The model under review builds one solid part; all positions refer to its coordinate system, in mm. Give positions to 0.01 mm unless a question says otherwise; leave off trailing zeros. Order: outer loops, then holes, each group sorted by start corner. A loop starts at its lowest first (then second) coordinate and runs counter-clockwise, first axis right, second up. Notation, with made-up numbers: (63.5, -6.5) - (110.5, -6.5) arc R31 cw to (110.5, 24.5) - close; hole circle Ø5 at (-14.75, 3.25). An arc over 180 degrees is marked (long way). Write item = value, one per line. Start each with the question number.
1. Mouldability with a two-part tool opening along X and no side actions: class faces 1 (the cylindrical face through (20.797, -14.859, 3.219)), 2 (the flat face through (0, 16, 3)), 3 (the cylindrical face through (-19.31, -13, 3.22)), 4 (the cylindrical face through (-20.859, 14.797, 3.219)) as pulls with the +X half, pulls with the -X half, needs draft (parallel to the pull), parting line crosses it, or undercut.
2. We need section B-B, the plane y = -6. Give the boundary of the cut face in (x, z), and give its area (3 significant figures).
3. We need section C-C, the plane y = -13. Give the boundary of the cut face in (x, z), and give its area (3 significant figures).
4. For P1, Ø2, axis at x = -9.19, y = -9.19, coming from the +Z side (3 decimals), flat-tipped, find the tip position at first contact; note if it passes through.
5. Wall thickness on probe 1 along Y at (x, z) = (18, 3.5); probe 2 along X at (y, z) = (11.5, 3); probe 3 along X at (y, z) = (-8.5, 2.5): over which ranges is each line inside the solid? List them lowest first.
6. We need section A-A, the plane x = 0. Give the boundary of the cut face in (y, z), and give its area (4 significant figures).
7. We need section D-D, the plane x = -9. Give the boundary of the cut face in (y, z).
from build123d import *

# Parameters (mm, degrees)
SKETCH1_W           = 44
SKETCH1_H           = 32
SKETCH1_R           = 9.5
SKETCH1_R_2         = 1.65
BOSS_EXTRUDE1_DEPTH = 6.35
SKETCH2_R           = 1.65
CUT_EXTRUDE1_DEPTH  = 28.934253167
FILLET1_R           = 4


with BuildPart() as part:
    # Sketch1 → Boss-Extrude1 (new body)
    with BuildSketch(Plane.XY):
        Rectangle(SKETCH1_W, SKETCH1_H)
        Circle(SKETCH1_R, mode=Mode.SUBTRACT)
        with Locations((-9.192388155, 9.192388155)):
            Circle(SKETCH1_R_2, mode=Mode.SUBTRACT)
        with Locations((9.192388155, 9.192388155)):
            Circle(SKETCH1_R_2, mode=Mode.SUBTRACT)
        with Locations((9.192388155, -9.192388155)):
            Circle(SKETCH1_R_2, mode=Mode.SUBTRACT)
        with Locations((-9.192388155, -9.192388155)):
            Circle(SKETCH1_R_2, mode=Mode.SUBTRACT)
    extrude(amount=BOSS_EXTRUDE1_DEPTH)

    # Sketch2 → Cut-Extrude1 (cut, through all)
    with BuildSketch(Plane.XY.offset(6.35)):
        with Locations((-18, 12)):
            Circle(SKETCH2_R)
        with Locations((-18, -12)):
            Circle(SKETCH2_R)
        with Locations((18, -12)):
            Circle(SKETCH2_R)
        with Locations((18, 12)):
            Circle(SKETCH2_R)
    extrude(amount=-CUT_EXTRUDE1_DEPTH, mode=Mode.SUBTRACT)

    # Fillet1
    fillet1_edges = [part.edges().sort_by_distance(p)[0] for p in [
        (-22, 16, 3.175),
        (22, 16, 3.175),
        (22, -16, 3.175),
        (-22, -16, 3.175),
    ]]
    fillet(fillet1_edges, radius=FILLET1_R)


solid = part.part
Model answer:
q1.face_1 = pulls with the +X half
q1.face_2 = needs draft
q1.face_3 = undercut
q1.face_4 = pulls with the -X half
q2.outline = (-22, 0) - (-7.37, 0) - (-7.37, 6.35) - (-22, 6.35) - close; (7.37, 0) - (22, 0) - (22, 6.35) - (7.37, 6.35) - close
q2.area = 186 mm2
q3.outline = (-21.87, 0) - (-19.31, 0) - (-19.31, 6.35) - (-21.87, 6.35) - close; (-16.69, 0) - (16.69, 0) - (16.69, 6.35) - (-16.69, 6.35) - close; (19.31, 0) - (21.87, 0) - (21.87, 6.35) - (19.31, 6.35) - close
q3.area = 244 mm2
q4.P1 = through
q5.probe_1 = -16 to -13.65, -10.35 to 10.35, 13.65 to 16
q5.probe_2 = -22 to -19.57, -16.43 to 16.43, 19.57 to 22
q5.probe_3 = -22 to -10.69, -7.69 to -4.24, 4.24 to 7.69, 10.69 to 22
q6.outline = (-16, 0) - (-9.5, 0) - (-9.5, 6.35) - (-16, 6.35) - close; (9.5, 0) - (16, 0) - (16, 6.35) - (9.5, 6.35) - close
q6.area = 82.55 mm2
q7.outline = (-16, 0) - (-10.83, 0) - (-10.83, 6.35) - (-16, 6.35) - close; (-7.55, 0) - (-3.04, 0) - (-3.04, 6.35) - (-7.55, 6.35) - close; (3.04, 0) - (7.55, 0) - (7.55, 6.35) - (3.04, 6.35) - close; (10.83, 0) - (16, 0) - (16, 6.35) - (10.83, 6.35) - close
